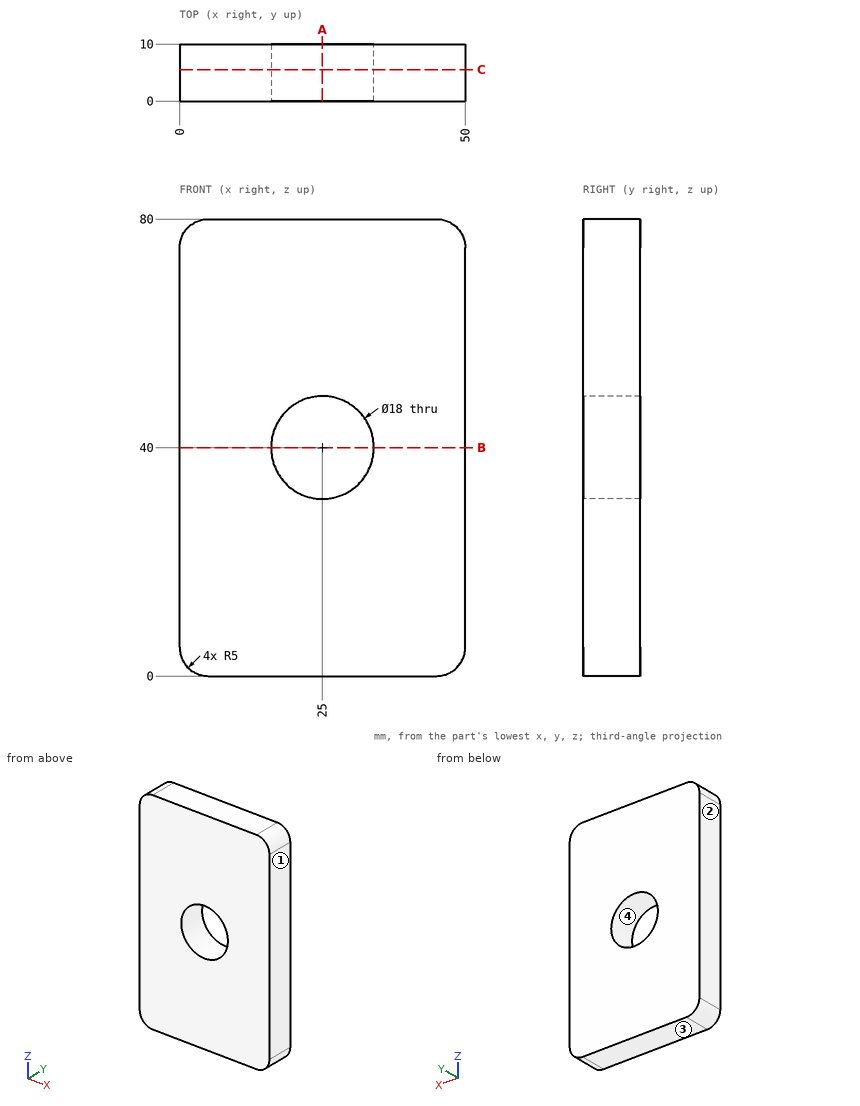
Verification items for this drawing (mm, ordinates from the low corner). Give positions to 0.01 mm unless a question says otherwise; leave off trailing zeros. Loops run counter-clockwise (first coordinate to the right, second up) from the corner with the lowest first, then second, coordinate; pieces in that order, holes last. Notation, with made-up numbers: M 68.5,48 L 112.5,48 A17 ccw 112.5,76 Z; hole C -21.75,18 d2. An arc over 180 degrees is marked long. Write each question's results on one line, items separated by ' | '.
1) Section check C-C, the plane y = 5.5. Record the boundary of the cut face in (x, z), plus the area to 3 significant figures.
Answers follow:
outline: M 0,5 A5 ccw 5,0 L 45,0 A5 ccw 50,5 L 50,75 A5 ccw 45,80 L 5,80 A5 ccw 0,75 Z; hole C 25,40 d18 | area: 3,720 mm2
2) Section check A-A, the plane x = 25. Record the boundary of the cut face in (y, z), plus the area to 3 significant figures.
Answers follow:
outline: M 0,0 L 10,0 L 10,31 L 0,31 Z; M 0,49 L 10,49 L 10,80 L 0,80 Z | area: 620 mm2
3) Thickness scan on line 1 (Z direction, x = 25, y = 7); line 2 (Z direction, x = 18.5, y = 8.5); line 3 (X direction, y = 6.25, z = 47). Record the ranges inside material, lowest first.
Answers follow:
line 1: 0 to 31, 49 to 80 | line 2: 0 to 33.78, 46.22 to 80 | line 3: 0 to 19.34, 30.66 to 50
4) Section check B-B, the plane z = 40. Record the boundary of the cut face in (x, y).
Answers follow:
outline: M 0,0 L 16,0 L 16,10 L 0,10 Z; M 34,0 L 50,0 L 50,10 L 34,10 Z
5) Gauge pin test, flat end, axial feed: pin 1 (1.5 mm diameter, centred on x = 21, y = 6, fed in from -Z). Record the tip position at first contact, or that the pin passes through.
Answers follow:
pin 1: z = 0
6) Release check for a two-part mould opening along X. For the marked faces 1, 2, 3 and 4 record: +X half, -X half, draft (parallel to the pull), parting line (faces both ways), or undercut.
Answers follow:
face 1: +X half | face 2: -X half | face 3: draft | face 4: undercut
